Print and shaded views of the part. All mm, measured from the part's lowest x, y and z. A direction names the side the tool comes from. Give positions to 0.01 mm unless a question says otherwise; leave off trailing zeros. Order: outer loops, then holes, each group sorted by start corner. A loop starts at its lowest first (then second) coordinate and runs counter-clockwise, first axis right, second up. Notation, with made-up numbers: (-38.75, 81) -> (-14.75, 81) arc R22 ccw to (-14.75, 113) -> close; hole circle Ø8 at (14.5, -39). An arc over 180 degrees is marked (long way). One line per question, with ' | ' between items. Start each with the question number.
(1) Cut at C-C (x = 12). Give the cut face in (y, z), then the cut area to 4 significant figures.
(2) Pull direction X, two halves, no side cores. Call the marked faces 1, 2, 3 and 4: +X half, -X half, draft (parallel to the pull), parting line (faces both ways), or undercut.
(3) Cut at B-B (z = 12). Give the cut face in (x, y).
(4) Drill centre lines: L1, parallel to Z at x = 12, y = 1.35; L2, parallel to Z at x = 12, y = 4.25. Where is each one in solid material? Low to high. Write a range as from..to.
(5) Cut at A-A (y = 2.5). Give the cut face in (x, z), then the cut area to 3 significant figures.
(6) Pin check, flat tips, straight feed: pin 1 Ø8 at (x, z) = (12, 12) entering from +Y; pin 2 Ø1.2 at (y, z) = (10, 2.5) entering from +X; pin 3 Ø5 at (x, z) = (26.5, 23) entering from +Y. Stop position of each tip, or through.
(7) Cut at D-D (x = 2.25). Give the cut face in (y, z).
(8) Which spindle directions (+Z, -Z, +X, -X, +Y, -Y) get a long thin tool onto all of the face, cutting with end or side? Do the marked faces 5, 6, 7 and 8. Say none if no direction does.
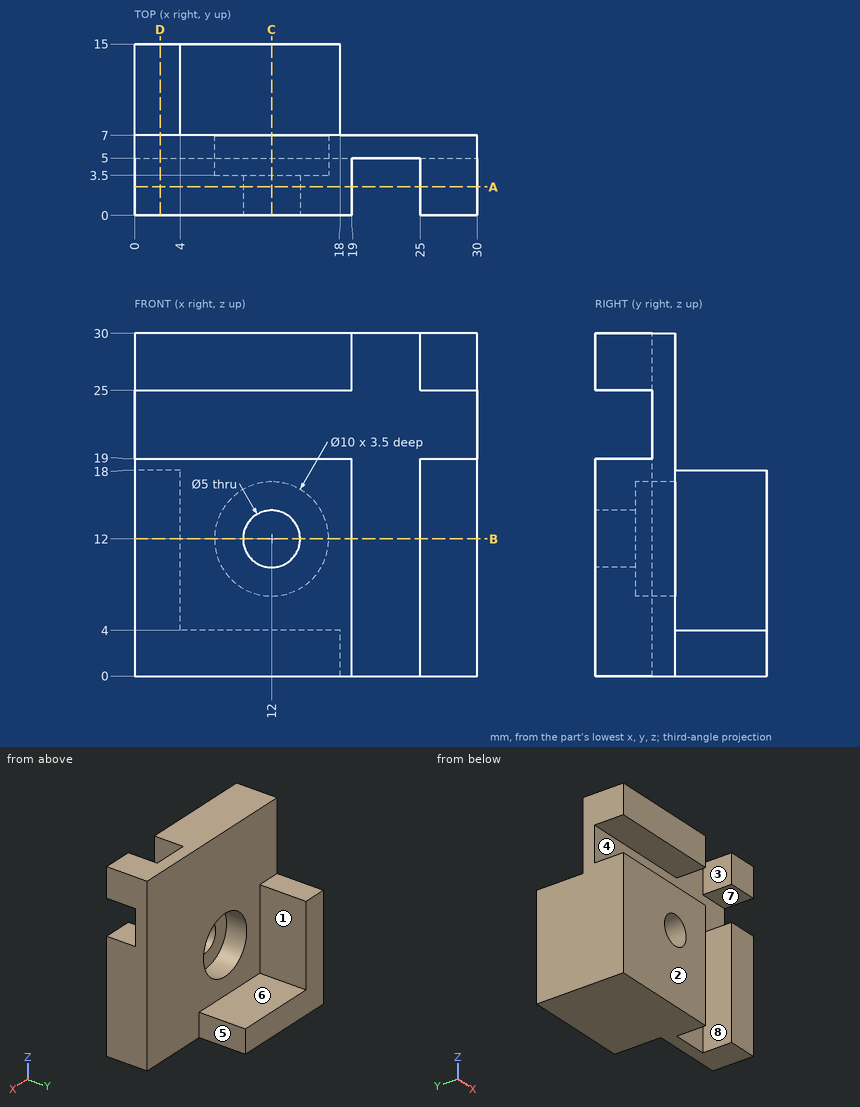
Result set:
1) outline: (0, 0) -> (15, 0) -> (15, 4) -> (7, 4) -> (7, 7) -> (3.5, 7) -> (3.5, 9.5) -> (0, 9.5) -> close; (0, 14.5) -> (3.5, 14.5) -> (3.5, 17) -> (7, 17) -> (7, 30) -> (0, 30) -> (0, 25) -> (5, 25) -> (5, 19) -> (0, 19) -> close | area: 159.5 mm2
2) face 1: +X half | face 2: draft | face 3: undercut | face 4: undercut
3) outline: (0, 0) -> (9.5, 0) -> (9.5, 3.5) -> (7, 3.5) -> (7, 7) -> (4, 7) -> (4, 15) -> (0, 15) -> close; (14.5, 0) -> (19, 0) -> (19, 5) -> (25, 5) -> (25, 0) -> (30, 0) -> (30, 7) -> (17, 7) -> (17, 3.5) -> (14.5, 3.5) -> close
4) L1: z = 0..9.5, 14.5..19, 25..30 | L2: z = 0..7, 17..19, 25..30
5) outline: (0, 0) -> (19, 0) -> (19, 19) -> (0, 19) -> close; (0, 25) -> (19, 25) -> (19, 30) -> (0, 30) -> close; (25, 0) -> (30, 0) -> (30, 19) -> (25, 19) -> close; (25, 25) -> (30, 25) -> (30, 30) -> (25, 30) -> close; hole circle Ø5 at (12, 12) | area: 556 mm2
6) pin 1: stops at y = 3.5 | pin 2: stops at x = 18 | pin 3: stops at y = 7
7) outline: (0, 0) -> (15, 0) -> (15, 18) -> (7, 18) -> (7, 30) -> (0, 30) -> (0, 25) -> (5, 25) -> (5, 19) -> (0, 19) -> close
8) face 5: +Z, -Z, +X, +Y | face 6: +Z, +X, +Y | face 7: +X, -X, -Y | face 8: +Z, -Z, -Y
